from build123d import *

# Parameters (mm, degrees)
SKETCH1_W           = 50.8
SKETCH1_H           = 25.4
SKETCH1_W_2         = 44.45
SKETCH1_H_2         = 19.05
EXTRUDE_THIN1_DEPTH = 19.05
SKETCH2_W           = 31.75
SKETCH2_H           = 3.175
BOSS_EXTRUDE1_DEPTH = 44.45
CUT_EXTRUDE1_REACH  = 55.975
SKETCH3_R           = 4.7625
CUT_EXTRUDE2_REACH  = 27.4
SKETCH4_R           = 1.5875
SKETCH8_R           = 3.175
CUT_EXTRUDE4_DEPTH  = 3.175


with BuildPart() as part:
    # Sketch1 → Extrude-Thin1 (new body, symmetric)
    with BuildSketch(Plane(origin=(0, 0, 0), x_dir=(0, 0, -1), z_dir=(1, 0, 0))):
        Rectangle(SKETCH1_W, SKETCH1_H)
        Rectangle(SKETCH1_W_2, SKETCH1_H_2, mode=Mode.SUBTRACT)
    extrude(amount=EXTRUDE_THIN1_DEPTH, both=True)

    # Sketch2 → Boss-Extrude1 (add)
    with BuildSketch(Plane.XZ.offset(12.7)):
        with Locations((0, 26.9875)):
            Rectangle(SKETCH2_W, SKETCH2_H)
    extrude(amount=-BOSS_EXTRUDE1_DEPTH)

    # Sketch3 → Cut-Extrude1 (cut, up to next)
    with BuildSketch(Plane.XY.offset(28.575), mode=Mode.PRIVATE) as cut_extrude1_sk1:
        with Locations((0, 22.225)):
            Circle(SKETCH3_R)
    cut_extrude1_tool1 = extrude(cut_extrude1_sk1.sketch, amount=-CUT_EXTRUDE1_REACH, mode=Mode.PRIVATE) & part.part
    add(cut_extrude1_tool1.solids().sort_by_distance((0, 22.225, 28.575))[0], mode=Mode.SUBTRACT)

    # Sketch4 → Cut-Extrude2 (cut, up to next)
    with BuildSketch(Plane(origin=(0, 12.7, 0), x_dir=(1, 0, 0), z_dir=(0, 1, 0)), mode=Mode.PRIVATE) as cut_extrude2_sk1:
        with Locations((14.2875, 3.175)):
            Circle(SKETCH4_R)
    cut_extrude2_tool1 = extrude(cut_extrude2_sk1.sketch, amount=-CUT_EXTRUDE2_REACH, mode=Mode.PRIVATE) & part.part
    add(cut_extrude2_tool1.solids().sort_by_distance((14.2875, 12.7, -3.175))[0], mode=Mode.SUBTRACT)
    # Sketch4 → Cut-Extrude2 (cut, up to next)
    with BuildSketch(Plane(origin=(0, 12.7, 0), x_dir=(1, 0, 0), z_dir=(0, 1, 0)), mode=Mode.PRIVATE) as cut_extrude2_sk2:
        with Locations((-14.2875, 3.175)):
            Circle(SKETCH4_R)
    cut_extrude2_tool2 = extrude(cut_extrude2_sk2.sketch, amount=-CUT_EXTRUDE2_REACH, mode=Mode.PRIVATE) & part.part
    add(cut_extrude2_tool2.solids().sort_by_distance((-14.2875, 12.7, -3.175))[0], mode=Mode.SUBTRACT)

    # Sketch8 → Cut-Extrude4 (cut)
    with BuildSketch(Plane.XZ.offset(12.7)):
        with Locations((0, -11.43)):
            Circle(SKETCH8_R)
        with Locations((0, 11.43)):
            Circle(SKETCH8_R)
    extrude(amount=-CUT_EXTRUDE4_DEPTH, mode=Mode.SUBTRACT)


solid = part.part
Geometry check sheet. Reference: the model listing, model coordinates, mm. A direction names the side the tool comes from. Round coordinates to 2 decimals unless told otherwise and drop trailing zeros. Order: outer loops, then holes, each group sorted by start corner. A loop starts at its lowest first (then second) coordinate and runs counter-clockwise, first axis right, second up. Notation, with made-up numbers: (62, 69.25) - (91, 69.25) arc R18 cw to (91, 86.25) - close; hole circle Ø1 at (47.25, 85.5). An arc over 180 degrees is marked (long way). One line per question, with ' | ' between items. Start each with the question number.
(1) Sectioned sample at A-A on x = 0. Count the separate pieces of the cut face and the enclosed holes in it, and give its area (3 significant figures).
(2) Depth check by flat-ended pin: pin 1 Ø21 at (x, y) = (-3.5, 24) entering from -Z; pin 2 Ø4 at (x, z) = (7, -8.5) entering from +Y; pin 3 Ø1 at (x, y) = (18, 2) entering from +Z. Enter the tip coordinate at first touch or a pass-through.
(3) Access from +Z, -Z, +X, -X, +Y, -Y to the whole of each face (thin tool, end or side, straight path). Record for faces 1 (the cylindrical face through (-0.41, -11.13, -8.28)), 2 (the flat face through (-15.875, 9, 27)), 3 (the cylindrical face through (-14.49, 11.13, -4.75)), 4 (the flat face through (0, 9.525, 0)).
(4) Thickness scan on L1, parallel to Z at x = 2, y = -7 (3 decimals); L2, parallel to Y at x = 7.5, z = -21.5 (3 decimals); L3, parallel to Z at x = 0, y = -10 (3 decimals). Record the ranges inside material, lowest first. Write a range as [from, to].
(5) Sectioned sample at B-B on z = 4.5. Record the cut outline in (x, y) (3 decimals), and give its area (3 significant figures).
(6) Release check for a two-part mould opening along Z. For faces 5 (the flat face through (3.3, 26.3, 25.4)), 6 (the flat face through (0, 12.7, 0)), 7 (the cylindrical face through (13.12, 11.13, -4.25)) record: released by +Z, released by -Z, zero draft, split by the parting line, or undercut.
(7) Sectioned sample at D-D on x = -17. Record the cut outline in (y, z) (3 decimals).
Conclusion:
1) separate pieces: 3 | enclosed holes: 0 | area: 514 mm2
2) pin 1: stops at z = 25.4 | pin 2: stops at y = 12.7 | pin 3: stops at z = 25.4
3) face 1: -Y | face 2: +Z, -X, +Y, -Y | face 3: +Y | face 4: +X, -X
4) L1: z = [-25.4, -22.225], [22.225, 28.575] | L2: y = [-12.7, -9.525], [9.525, 12.7] | L3: z = [-25.4, -14.605], [-8.255, 8.255], [14.605, 28.575]
5) outline: (-19.05, -12.7) - (19.05, -12.7) - (19.05, -9.525) - (-19.05, -9.525) - close; (-19.05, 9.525) - (19.05, 9.525) - (19.05, 12.7) - (-19.05, 12.7) - close | area: 242 mm2
6) face 5: released by -Z | face 6: zero draft | face 7: undercut
7) outline: (-12.7, -25.4) - (12.7, -25.4) - (12.7, 25.4) - (-12.7, 25.4) - close; hole (-9.525, -22.225) - (9.525, -22.225) - (9.525, 22.225) - (-9.525, 22.225) - close
